Geometry: final body of the model. Coordinates: model frame, mm. A direction names the side the tool comes from. Give positions to 0.01 mm unless a question says otherwise; leave off trailing zeros. Loops run counter-clockwise (first coordinate to the right, second up) from the corner with the lowest first, then second, coordinate; pieces in that order, holes last. Notation, with made-up numbers: (59.25, 77.25) -> (117.25, 77.25) arc R17 ccw to (117.25, 106.25) -> close; hole circle Ø1 at (51, 14.25). An arc over 180 degrees is marked (long way). Answer in a Markdown table with one row per item. Add a question column.
from build123d import *

# Parameters (mm, degrees)
BOSS_EXTRU_1_DEPTH      = 130
ESQUISSE4_R             = 54.250129783
ESQUISSE4_R_2           = 27.5
ENL_V_MAT_EXTRU_1_DEPTH = 150.53980461
ESQUISSE5_R             = 10
ESQUISSE5_R_2           = 3
ENL_V_MAT_EXTRU_2_DEPTH = 136.114727886
BOSS_EXTRU_2_DEPTH      = 5
ESQUISSE6_R             = 2
ENL_V_MAT_EXTRU_3_DEPTH = 140.046443052
BOSS_EXTRU_3_DEPTH      = 49.27879
ENL_V_START             = -8.6
ESQUISSE9_W             = 6.5
ESQUISSE9_H             = 35.278790482
ESQUISSE9_W_2           = 18
ESQUISSE9_H_2           = 40.466483264
ENL_V_MAT_EXTRU_4_DEPTH = 8.6


with BuildPart() as part:
    # Esquisse1 → Boss.-Extru.1 (new body)
    with BuildSketch(Plane.XY):
        with BuildLine():
            Line((-18, -51.176914536), (-18, -48.176914536))
            ThreePointArc((-18, -48.176914536), (-9.5, -16.454482672), (-32.722431864, -39.676914536))
            Line((-32.722431864, -39.676914536), (-35.320508076, -41.176914536))
            ThreePointArc((-35.320508076, -41.176914536), (-37.98683472, -30.451354144), (-34.549834435, -19.947356212))
            ThreePointArc((-34.549834435, -19.947356212), (-45.365063628, -17.671886805), (-53.320508076, -10))
            Line((-53.320508076, -10), (-50.722431864, -8.5))
            ThreePointArc((-50.722431864, -8.5), (-19, 0), (-50.722431864, 8.5))
            Line((-50.722431864, 8.5), (-53.320508076, 10))
            ThreePointArc((-53.320508076, 10), (-45.365063628, 17.671886805), (-34.549834435, 19.947356212))
            ThreePointArc((-34.549834435, 19.947356212), (-37.98683472, 30.451354144), (-35.320508076, 41.176914536))
            Line((-35.320508076, 41.176914536), (-32.722431864, 39.676914536))
            ThreePointArc((-32.722431864, 39.676914536), (-9.5, 16.454482672), (-18, 48.176914536))
            Line((-18, 48.176914536), (-18, 51.176914536))
            ThreePointArc((-18, 51.176914536), (-7.378228908, 48.123240948), (0, 39.894712423))
            ThreePointArc((0, 39.894712423), (7.378228908, 48.123240948), (18, 51.176914536))
            Line((18, 51.176914536), (18, 48.176914536))
            ThreePointArc((18, 48.176914536), (9.5, 16.454482672), (32.722431864, 39.676914536))
            Line((32.722431864, 39.676914536), (35.320508076, 41.176914536))
            ThreePointArc((35.320508076, 41.176914536), (37.98683472, 30.451354144), (34.549834435, 19.947356212))
            ThreePointArc((34.549834435, 19.947356212), (45.365063628, 17.671886805), (53.320508076, 10))
            Line((53.320508076, 10), (50.722431864, 8.5))
            ThreePointArc((50.722431864, 8.5), (19, 0), (50.722431864, -8.5))
            Line((50.722431864, -8.5), (53.320508076, -10))
            ThreePointArc((53.320508076, -10), (45.365063628, -17.671886805), (34.549834435, -19.947356212))
            ThreePointArc((34.549834435, -19.947356212), (37.98683472, -30.451354144), (35.320508076, -41.176914536))
            Line((35.320508076, -41.176914536), (32.722431864, -39.676914536))
            ThreePointArc((32.722431864, -39.676914536), (9.5, -16.454482672), (18, -48.176914536))
            Line((18, -48.176914536), (18, -51.176914536))
            ThreePointArc((18, -51.176914536), (7.378228908, -48.123240948), (0, -39.894712423))
            ThreePointArc((0, -39.894712423), (-7.378228908, -48.123240948), (-18, -51.176914536))
        make_face()
    extrude(amount=BOSS_EXTRU_1_DEPTH)

    # Esquisse4 → Enlèv. mat.-Extru.1 (cut, through all)
    with BuildSketch(Plane.XY.offset(130)):
        Circle(ESQUISSE4_R)
        Circle(ESQUISSE4_R_2, mode=Mode.SUBTRACT)
    extrude(amount=-ENL_V_MAT_EXTRU_1_DEPTH, mode=Mode.SUBTRACT)

    # Esquisse5 → Enlèv. mat.-Extru.2 (cut, through all)
    with BuildSketch(Plane.XY.offset(130)):
        Circle(ESQUISSE5_R)
        with Locations((0, 15)):
            Circle(ESQUISSE5_R_2)
        with Locations((12.990381057, 7.5)):
            Circle(ESQUISSE5_R_2)
        with Locations((12.990381057, -7.5)):
            Circle(ESQUISSE5_R_2)
        with Locations((0, -15)):
            Circle(ESQUISSE5_R_2)
        with Locations((-12.990381057, 7.5)):
            Circle(ESQUISSE5_R_2)
        Polygon((14.206088614, -14.605667257), (5.545834576, -19.605667257), (4.695834576, -18.13342407), (13.356088614, -13.13342407), align=None)
        Polygon((18.051923191, 5), (19.751923191, 5), (19.751923191, -5), (18.051923191, -5), (18.051923191, -1.5), (14.051923191, -1.5), (14.051923191, 1.5), (18.051923191, 1.5), align=None)
        Polygon((-14.206088614, 14.605667257), (-5.545834576, 19.605667257), (-4.695834576, 18.13342407), (-13.356088614, 13.13342407), align=None)
        Polygon((5.545834576, 19.605667257), (14.206088614, 14.605667257), (13.356088614, 13.13342407), (4.695834576, 18.13342407), align=None)
        Polygon((0.986461417, -27.708601295), (-23.503121916, 14.708601295), (-40.823629992, 4.708601295), (-16.334046658, -37.708601295), align=None)
    extrude(amount=-ENL_V_MAT_EXTRU_2_DEPTH, mode=Mode.SUBTRACT)

    # Esquisse7 → Boss.-Extru.2 (add)
    with BuildSketch(Plane(origin=(-11.258330249, -6.5, 0), x_dir=(0, 0, 1), z_dir=(-0.8660254037844403, -0.49999999999999717, 0))):
        Polygon((8, 24.233241632), (0, 24.233241632), (0, 32.233241632), (-10, 32.233241632), (-10, -32.233241632), (0, -32.233241632), (0, -24.233241632), (8, -24.233241632), align=None)
    extrude(amount=BOSS_EXTRU_2_DEPTH)

    # Esquisse6 → Enlèv. mat.-Extru.3 (cut, through all)
    with BuildSketch(Plane(origin=(-11.258330249, -6.5, 0), x_dir=(0, 0, 1), z_dir=(-0.8660254037844403, -0.49999999999999717, 0))):
        with Locations(Location((-4, 28, 0), (0, 0, 270))):
            Circle(ESQUISSE6_R)
        with Locations(Location((-4, -28, 0), (0, 0, 90))):
            Circle(ESQUISSE6_R)
    extrude(amount=ENL_V_MAT_EXTRU_3_DEPTH, mode=Mode.SUBTRACT)

    # Esquisse8 → Boss.-Extru.3 (add)
    with BuildSketch(Plane(origin=(12.116620816, -20.986602869, 0), x_dir=(0.8660254037844403, 0.4999999999999971, 0), z_dir=(0.49999999999999717, -0.8660254037844404, 0))):
        Polygon((-13, 130), (-21.6, 130), (-21.6, 123.5), (-19.6, 123.5), (-19.6, 125.5), (-18, 125.5), (-18, 123.5), (-13, 123.5), align=None)
    extrude(amount=-BOSS_EXTRU_3_DEPTH)

    # Esquisse9 → Enlèv. mat.-Extru.4 (cut)
    with BuildSketch(Plane(origin=(-18.706148722, -10.8, 0), x_dir=(0, 0, 1), z_dir=(-0.8660254037844403, -0.49999999999999734, 0)).offset(ENL_V_START)):
        with Locations((126.75, 0.406153609)):
            Rectangle(ESQUISSE9_W, ESQUISSE9_H)
        with Locations((-1, 0)):
            Rectangle(ESQUISSE9_W_2, ESQUISSE9_H_2)
    extrude(amount=ENL_V_MAT_EXTRU_4_DEPTH, mode=Mode.SUBTRACT)


solid = part.part
(1) Cut plane A-A on y = -7.5. Return the cut outline in (x, z).
(2) Draft query along X for faces 1 (the flat face through (1, -32, 0)), 2 (the flat face through (14.052, 0, 66)), 3 (the cylindrical face through (-2.17, -9.76, 65.91)). Return one class per face: +X half, -X half, draft (parallel to the pull), parting line (faces both ways), or undercut.
(3) Reachability of faces 4 (the flat face through (18.052, -3, 66)), 5 (the flat face through (-6.58, -27.8, 124.49)), 6 (the flat face through (-3.276, -25.255, -1.126)), 7 (the flat face through (-3.18, -30.49, -3.13)) from +Z, -Z, +X, -X, +Y, -Y: full face, straight path, thin tool, end or side. Return the list, or none.
(4) Cut plane B-B on z = 2.5. State how many separate pieces and enclosed holes the cut face has, then the cut area to 3 significant figures.
(5) Material intervals for line 1 along Y through (x, z) = (10.5, 8.5); line 2 along Y through (x, z) = (7.5, 65); line 3 along Y through (x, z) = (-8, 26.5), sorted ascending. Write a range as from..to.
(6) Pin query (flat end, axial travel): pin 1 Ø8.5 at (x, y) = (-4, -24) entering from -Z; pin 2 Ø1.6 at (x, y) = (-8, -29) entering from -Z; pin 3 Ø3 at (y, z) = (4, 58) entering from +X; pin 4 Ø1.5 at (x, z) = (-17.5, 13.5) entering from +Y. Return the tip coordinate at first contact, or that it passes through.
(7) Cut plane C-C on y = 0. Return the cut outline in (x, z), then the cut area to 3 significant figures.
Answer list:
| question | item | result |
|---|---|---|
| 1 | outline | (-10.68, 0) -> (-6.61, 0) -> (-6.61, 130) -> (-10.68, 130) -> close; (6.61, 0) -> (9.99, 0) -> (9.99, 130) -> (6.61, 130) -> close; (15.99, 0) -> (20.74, 0) -> (20.74, 130) -> (15.99, 130) -> close |
| 2 | face 1 | draft |
| 2 | face 2 | +X half |
| 2 | face 3 | undercut |
| 3 | face 4 | +Z, -Z, +X |
| 3 | face 5 | -Z |
| 3 | face 6 | -Z, -X |
| 3 | face 7 | -Z, -X, -Y |
| 4 | separate pieces | 1 |
| 4 | enclosed holes | 6 |
| 4 | area | 817 mm² |
| 5 | line 1 | y = -14.78..-9.17, -5.83..5.83, 9.17..14.78 |
| 5 | line 2 | y = -16.51..-6.61, 6.61..16.51 |
| 5 | line 3 | y = -12.14..-6, 6..16.23 |
| 6 | pin 1 | stops at z = -10 |
| 6 | pin 2 | stops at z = 123.5 |
| 6 | pin 3 | stops at x = 19.91 |
| 6 | pin 4 | stops at y = 14.22 |
| 7 | outline | (-15.01, 0) -> (-10, 0) -> (-10, 130) -> (-15.01, 130) -> close; (10, 0) -> (14.05, 0) -> (14.05, 130) -> (10, 130) -> close |
| 7 | area | 1,180 mm² |
